from build123d import *

# Parameters (mm, degrees)
F1_DEPTH = 2


with BuildPart() as f1:
    # F0 (on Front) → F1 (new body, symmetric)
    with BuildSketch(Plane.XZ):
        with BuildLine():
            Line((20.67841, 3), (0, 3))
            Line((0, 3), (-20.67841, 3))
            ThreePointArc((-20.67841, 3), (-24.719861, 3.59602), (-28.417201, 5.333333))
            ThreePointArc((-28.417201, 5.333333), (-35.019592, 8.435678), (-42.236471, 9.5))
            Line((-42.236471, 9.5), (-57.5, 9.5))
            Line((-57.5, 9.5), (-57.5, -9.5))
            Line((-57.5, -9.5), (-42.236471, -9.5))
            ThreePointArc((-42.236471, -9.5), (-35.019592, -8.435678), (-28.417201, -5.333333))
            ThreePointArc((-28.417201, -5.333333), (-24.719861, -3.59602), (-20.67841, -3))
            Line((-20.67841, -3), (0, -3))
            Line((0, -3), (20.67841, -3))
            ThreePointArc((20.67841, -3), (24.719861, -3.59602), (28.417201, -5.333333))
            ThreePointArc((28.417201, -5.333333), (35.019592, -8.435678), (42.236471, -9.5))
            Line((42.236471, -9.5), (57.5, -9.5))
            Line((57.5, -9.5), (57.5, 9.5))
            Line((57.5, 9.5), (42.236471, 9.5))
            ThreePointArc((42.236471, 9.5), (35.019592, 8.435678), (28.417201, 5.333333))
            ThreePointArc((28.417201, 5.333333), (24.719861, 3.59602), (20.67841, 3))
        make_face()
    extrude(amount=F1_DEPTH, both=True)


solid = f1.part
Check sheet for the modelled part. Datum: model origin and axes. Units: mm. A direction names the side the tool comes from. Give positions to 0.01 mm unless a question says otherwise; leave off trailing zeros. Loops run counter-clockwise (first coordinate to the right, second up) from the corner with the lowest first, then second, coordinate; pieces in that order, holes last. Notation, with made-up numbers: M -19.75,-20.5 L -6.75,-20.5 A6 ccw -6.75,-16.5 Z; hole C 79.5,88 d2. An arc over 180 degrees is marked long. Use a Markdown table: item, result. Add a question column.
Q1. Sectioned sample at B-B, the plane x = 10. Record the cut outline in (y, z), then the cut area to 3 significant figures.
Q2. Sectioned sample at C-C, the plane x = -33. Record the cut outline in (y, z).
Q3. Tool access check on faces 5 (the flat face through (-1, 2, 0)), 6 (the flat face through (0, 0, 3)), 7 (the flat face through (0, 0, -3)). Record the directions out of +Z, -Z, +X, -X, +Y, -Y that give a thin tool (end or side, any length) a straight path to the whole face; none if there is none.
Q4. Scan lines: line 1 along Z through (x, y) = (12, -1.2); line 2 along X through (y, z) = (1.45, 6.75); line 3 along X through (y, z) = (-0.35, -7.5). Record each from-to range of solid material in increasing order. Write a range as [from, to].
Q5. Go/stop test with flat-tipped pins: pin 1 (2 mm diameter, centred on x = -12, y = 1, fed in from -Z); pin 2 (2 mm diameter, centred on x = -14.5, y = 0, fed in from +Z). Record where each tip stops, or that it passes through.
Q6. Sectioned sample at A-A, the plane y = 0.75. Record the cut outline in (x, z), then the cut area to 3 significant figures.
Q7. Mould release check, pull along X, two halves, no side actions. Record for faces 1 (the cylindrical face through (35.118, -0.028, 8.465)), 2 (the flat face through (-57.5, 0, 0)), 3 (the flat face through (50, 0, 9.5)), 4 (the cylindrical face through (-35.118, -0.028, -8.465)): pulls with the +X half, pulls with the -X half, needs draft (parallel to the pull), parting line crosses it, or undercut.
Verdict:
| question | item | result |
|---|---|---|
| 1 | outline | M -2,-3 L 2,-3 L 2,3 L -2,3 Z |
| 1 | area | 24.0 mm^2 |
| 2 | outline | M -2,-7.73 L 2,-7.73 L 2,7.73 L -2,7.73 Z |
| 3 | face 5 | +Z, -Z, +X, -X, +Y |
| 3 | face 6 | +Z, +Y, -Y |
| 3 | face 7 | -Z, +Y, -Y |
| 4 | line 1 | [-3, 3] |
| 4 | line 2 | [-57.5, -30.84], [30.84, 57.5] |
| 4 | line 3 | [-57.5, -32.44], [32.44, 57.5] |
| 5 | pin 1 | z = -3 |
| 5 | pin 2 | z = 3 |
| 6 | outline | M -57.5,-9.5 L -42.24,-9.5 A25 ccw -28.42,-5.33 A14 cw -20.68,-3 L 20.68,-3 A14 cw 28.42,-5.33 A25 ccw 42.24,-9.5 L 57.5,-9.5 L 57.5,9.5 L 42.24,9.5 A25 ccw 28.42,5.33 A14 cw 20.68,3 L -20.68,3 A14 cw -28.42,5.33 A25 ccw -42.24,9.5 L -57.5,9.5 Z |
| 6 | area | 1,400 mm^2 |
| 7 | face 1 | undercut |
| 7 | face 2 | pulls with the -X half |
| 7 | face 3 | needs draft |
| 7 | face 4 | undercut |
